Check sheet for the modelled part. Datum: model origin and axes. Units: mm. A direction names the side the tool comes from. Round coordinates to 2 decimals unless told otherwise and drop trailing zeros. Answer in a Markdown table with one row per item.
from build123d import *

# Parameters (mm, degrees)
SKETCH1_W                                = 1250
SKETCH1_H                                = 115
BOSS_EXTRUDE1_DEPTH                      = 35
CUT_EXTRUDE1_DEPTH                       = 70
CUT_EXTRUDE3_START                       = -70
SKETCH9_W                                = 25
SKETCH9_H                                = 38.657600419
CUT_EXTRUDE3_DEPTH                       = 70
LPATTERN1_COUNT                          = 9
LPATTERN1_PITCH                          = 133
LPATTERN2_COUNT                          = 9
LPATTERN2_PITCH                          = 133
LPATTERN2_COL_COUNT                      = 2
LPATTERN2_COL_PITCH                      = 133
LPATTERN3_COUNT                          = 7
LPATTERN3_PITCH                          = 133
CUT_EXTRUDE2_DEPTH                       = 7
M8_TAPPED_HOLE1_AT_2_COUNT               = 2
M8_TAPPED_HOLE1_AT_2_PITCH               = 66
CBORE_FOR_M20_HEX_HEAD_BOLT1_D           = 22
CBORE_FOR_M20_HEX_HEAD_BOLT1_CBORE_D     = 35
CBORE_FOR_M20_HEX_HEAD_BOLT1_CBORE_DEPTH = 72
LPATTERN4_COUNT                          = 3
LPATTERN4_PITCH                          = 525
SKETCH14_W                               = 22
SKETCH14_H                               = 70
CUT_EXTRUDE4_DEPTH                       = 7


with BuildPart() as part:
    # Sketch1 → Boss-Extrude1 (new, symmetric)
    with BuildSketch(Plane.XY):
        with Locations((0, 57.5)):
            Rectangle(SKETCH1_W, SKETCH1_H)
    extrude(amount=BOSS_EXTRUDE1_DEPTH, both=True)

    # Sketch2 → Cut-Extrude1 (cut)
    with BuildSketch(Plane.XY.offset(35)):
        Polygon((-475.945987185, 115), (-588.054012815, 115), (-567.86, 100.86), (-542, 75), (-542, 65), (-522, 65), (-522, 75), (-496.14, 100.86), align=None)
    cut_extrude1 = extrude(amount=-CUT_EXTRUDE1_DEPTH, mode=Mode.SUBTRACT)

    # Sketch9 → Cut-Extrude3 (cut)
    with BuildSketch(Plane.XY.offset(35).offset(CUT_EXTRUDE3_START)):
        with Locations((-532, 84.32880021)):
            Rectangle(SKETCH9_W, SKETCH9_H)
    cut_extrude3 = extrude(amount=CUT_EXTRUDE3_DEPTH, mode=Mode.SUBTRACT)

    # Sketch4 → M20 Tapped Hole1 (revolve, cut)
    with BuildSketch(Plane(origin=(-465.330987185, 115, 0), x_dir=(0, 0, 1), z_dir=(1, 0, 0))):
        Polygon((0, 0), (0, 45.257530416), (8.75, 40), (8.75, 0), align=None)
    m20_tapped_hole1 = revolve(axis=Axis((-465.330987185, 121.35, 0), (0, -1, 0)), mode=Mode.SUBTRACT)

    # LPattern1: Cut-Extrude1, Cut-Extrude3 ×9
    with Locations(*[(i * LPATTERN1_PITCH, 0, 0) for i in range(1, LPATTERN1_COUNT)]):
        add(cut_extrude1, mode=Mode.SUBTRACT)
        add(cut_extrude3, mode=Mode.SUBTRACT)

    # LPattern2: M20 Tapped Hole1 ×9
    with Locations(*[(i * LPATTERN2_PITCH, 0, 0) for i in range(1, LPATTERN2_COUNT)]):
        add(m20_tapped_hole1, mode=Mode.SUBTRACT)

    # LPattern2 col: M20 Tapped Hole1 ×2
    with Locations(*[(-i * LPATTERN2_COL_PITCH, 0, 0) for i in range(1, LPATTERN2_COL_COUNT)]):
        add(m20_tapped_hole1, mode=Mode.SUBTRACT)

    # Sketch7 → M20 Tapped Hole2 (revolve, cut)
    with BuildSketch(Plane(origin=(-399, 65, 0), x_dir=(0, 0, 1), z_dir=(1, 0, 0))):
        Polygon((0, 0), (0, 45.257530416), (8.75, 40), (8.75, 0), align=None)
    m20_tapped_hole2 = revolve(axis=Axis((-399, 71.35, 0), (0, -1, 0)), mode=Mode.SUBTRACT)

    # LPattern3: M20 Tapped Hole2 ×7, 1 skipped
    with Locations(*[(i * LPATTERN3_PITCH, 0, 0) for i in range(1, LPATTERN3_COUNT) if i not in (3,)]):
        add(m20_tapped_hole2, mode=Mode.SUBTRACT)

    # Sketch8 → Cut-Extrude2 (cut)
    with BuildSketch(Plane.XZ):
        with BuildLine():
            Line((-461, 35), (-439, 35))
            Line((-439, 35), (-439, 11))
            Line((-439, 11), (-350, 11))
            ThreePointArc((-350, 11), (-339, 0), (-350, -11))
            Line((-350, -11), (-439, -11))
            Line((-439, -11), (-439, -35))
            Line((-439, -35), (-461, -35))
            Line((-461, -35), (-461, 35))
        make_face()
    cut_extrude2 = extrude(amount=-CUT_EXTRUDE2_DEPTH, mode=Mode.SUBTRACT)

    # Sketch13 → M8 Tapped Hole1 (revolve, cut)
    with BuildSketch(Plane(origin=(-450, 7, 0), x_dir=(0, 0, -1), z_dir=(1, 0, 0))):
        Polygon((0, 0), (0, 22.042926105), (3.4, 20), (3.4, 0), align=None)
    m8_tapped_hole1 = revolve(axis=Axis((-450, 0.65, 0), (0, 1, 0)), mode=Mode.SUBTRACT)

    # M8 Tapped Hole1 at 2: M8 Tapped Hole1 ×2
    with Locations(*[(i * M8_TAPPED_HOLE1_AT_2_PITCH, 0, 0) for i in range(1, M8_TAPPED_HOLE1_AT_2_COUNT)]):
        add(m8_tapped_hole1, mode=Mode.SUBTRACT)

    # Mirror1: Cut-Extrude2, M8 Tapped Hole1 across plane
    add(cut_extrude2.mirror(Plane(origin=(0, 0, 0), x_dir=(0, 0, 1), z_dir=(1, 0, 0))), mode=Mode.SUBTRACT)
    add(m8_tapped_hole1.mirror(Plane(origin=(0, 0, 0), x_dir=(0, 0, 1), z_dir=(1, 0, 0))), mode=Mode.SUBTRACT)

    # Mirror1 copy 1 sketch → Mirror1 copy 1 (revolve, cut)
    with BuildSketch(Plane(origin=(384, 7, 0), x_dir=(0, 0, -1), z_dir=(-1, 0, 0))):
        Polygon((0, 0), (0, -22.042926105), (3.4, -20), (3.4, 0), align=None)
    revolve(axis=Axis((384, 0.65, 0), (0, -1, 0)), mode=Mode.SUBTRACT)

    # CBORE for M20 Hex Head Bolt1 (through all)
    with Locations(Plane(origin=(0, 115, 0), x_dir=(1, 0, 0), z_dir=(0, 1, 0))):
        with Locations((-525, 0)):
            cbore_for_m20_hex_head_bolt1 = CounterBoreHole(CBORE_FOR_M20_HEX_HEAD_BOLT1_D / 2, CBORE_FOR_M20_HEX_HEAD_BOLT1_CBORE_D / 2, CBORE_FOR_M20_HEX_HEAD_BOLT1_CBORE_DEPTH)

    # LPattern4: CBORE for M20 Hex Head Bolt1 ×3
    with Locations(*[(i * LPATTERN4_PITCH, 0, 0) for i in range(1, LPATTERN4_COUNT)]):
        add(cbore_for_m20_hex_head_bolt1, mode=Mode.SUBTRACT)

    # Sketch14 → Cut-Extrude4 (cut)
    with BuildSketch(Plane.XZ):
        Rectangle(SKETCH14_W, SKETCH14_H)
    extrude(amount=-CUT_EXTRUDE4_DEPTH, mode=Mode.SUBTRACT)


solid = part.part
Item 1: Mould release check, pull along X, two halves, no side actions. Record for faces 6 (the flat face through (195, 115, 8)), 7 (the flat face through (-625, 57, 0)), 8 (the flat face through (45.816, 107.831, 0.49)): pulls with the +X half, pulls with the -X half, needs draft (parallel to the pull), parting line crosses it, or undercut.
Result sheet:
| item | result |
|---|---|
| face 6 | needs draft |
| face 7 | pulls with the -X half |
| face 8 | undercut |
Item 2: Depth check by flat-ended pin: P1, Ø7, axis at x = -1, z = -23.5, coming from the +Y side; P2, Ø17.5, axis at x = -3.5, z = 2.5, coming from the +Y side; P3, Ø11, axis at x = -384, z = 0, coming from the +Y side. Enter the tip coordinate at first touch or a pass-through.
Result sheet:
| item | result |
|---|---|
| P1 | stops at y = 65 |
| P2 | stops at y = 43 |
| P3 | stops at y = 85.5 |
Item 3: Set-up check for faces 1 (the flat face through (0, 7, -21)), 2 (the flat face through (-8, 43, 8)), 3 (the flat face through (-290, 89, 0)), 4 (the flat face through (461, 115, 8)), 5 (the flat face through (625, 57, 0)): record each of +Z, -Z, +X, -X, +Y, -Y from which the full face is reachable in a straight line by a thin tool's end or side.
Result sheet:
| item | result |
|---|---|
| face 1 | +Z, -Z, -Y |
| face 2 | +Y |
| face 3 | +Z, -Z, +Y |
| face 4 | +Z, -Z, +X, -X, +Y |
| face 5 | +Z, -Z, +X, +Y, -Y |
Item 4: Scan lines: line 1 (Z direction, x = 0, y = 63.5); line 2 (Z direction, x = 266, y = 38); line 3 (Y direction, x = 410.5, z = 10). Record each from-to range of solid material in increasing order. Write a range as [from, to].
Result sheet:
| item | result |
|---|---|
| line 1 | z = [-35, -17.5], [17.5, 35] |
| line 2 | z = [-35, -8.75], [8.75, 35] |
| line 3 | y = [7, 65] |
